Source: CAD feature listing. Evaluate the final solid. Frame: model axes, mm. A direction names the side the tool comes from. Coordinates: 2 decimals unless noted, no trailing zeros. Write each loop counter-clockwise with the first axis right and the second up, starting at its lowest first coordinate (ties: lowest second). Pieces come first, ordered by that corner, then holes. Notation, with made-up numbers: (-28, 4) - (-10, 4) arc R34 ccw to (-10, 35) - close; hole circle Ø9 at (81.5, 82.25). An arc over 180 degrees is marked (long way). One line per question, with ' | ' between items.
from build123d import *

# Parameters (mm, degrees)
F0_W     = 60
F0_H     = 20
F0_R     = 2.5
F1_DEPTH = 4
F2_W     = 20
F2_H     = 69
F2_R     = 2.5
F3_DEPTH = 4
F5_DEPTH = 60
F7_DEPTH = 65


with BuildPart() as f1:
    # F0 (on Top) → F1 (new body)
    with BuildSketch(Plane.XY):
        with Locations((30, 10)):
            Rectangle(F0_W, F0_H)
        with Locations((10, 10)):
            Circle(F0_R, mode=Mode.SUBTRACT)
        with Locations((30, 10)):
            Circle(F0_R, mode=Mode.SUBTRACT)
        with Locations((50, 10)):
            Circle(F0_R, mode=Mode.SUBTRACT)
    extrude(amount=F1_DEPTH)

    # F2 (on Right) → F3 (join)
    with BuildSketch(Plane.YZ):
        with Locations((10, 34.5)):
            Rectangle(F2_W, F2_H)
        with Locations((10, 14)):
            Circle(F2_R, mode=Mode.SUBTRACT)
        with Locations((10, 34)):
            Circle(F2_R, mode=Mode.SUBTRACT)
        with Locations((10, 54)):
            Circle(F2_R, mode=Mode.SUBTRACT)
    extrude(amount=-F3_DEPTH)

    # F4 (on face) → F5 (join, through all)
    with BuildSketch(Plane.YZ.offset(60)):
        Polygon((7, 5.5), (5.5, 4), (14.5, 4), (13, 5.5), align=None)
    extrude(amount=-F5_DEPTH)

    # F6 (on face) → F7 (join, through all)
    with BuildSketch(Plane.XY.offset(69)):
        Polygon((1.5, 13), (0, 14.5), (0, 5.5), (1.5, 7), align=None)
    extrude(amount=-F7_DEPTH)


solid = f1.part
Item 1: Cut plane A-A on x = 13.5. Return loops of the section in (y, z), and give its area (4 significant figures).
Check sheet entries:
outline: (0, 0) - (20, 0) - (20, 4) - (14.5, 4) - (13, 5.5) - (7, 5.5) - (5.5, 4) - (0, 4) - close | area: 91.25 mm²
Item 2: Pin query (flat end, axial travel): pin 1 Ø3 at (x, y) = (10, 10) entering from -Z; pin 2 Ø3 at (y, z) = (3, 27) entering from +X; pin 3 Ø8 at (x, y) = (30, 10) entering from +Z. Return the tip coordinate at first contact, or that it passes through.
Check sheet entries:
pin 1: z = 4 | pin 2: x = 0 | pin 3: z = 5.5
Item 3: Cut plane C-C on y = 15.75. Return loops of the section in (x, z), and give its area (3 significant figures).
Check sheet entries:
outline: (-4, 0) - (60, 0) - (60, 4) - (0, 4) - (0, 69) - (-4, 69) - close | area: 516 mm²
Item 4: Mould query, pull axis Z, two halves, no side actions, for faces 1 (the face through (52.31, 9.04, 1.97)), 2 (the face through (30, 3, 4)), 3 (the face through (-1.97, 9.46, 11.56)). Classes: pulls with the +Z half, pulls with the -Z half, needs draft (parallel to the pull), parting line crosses it, or undercut.
Check sheet entries:
face 1: needs draft | face 2: pulls with the +Z half | face 3: undercut
Item 5: Cut plane B-B on z = 30. Return loops of the section in (x, y).
Check sheet entries:
outline: (-4, 0) - (0, 0) - (0, 5.5) - (1.5, 7) - (1.5, 13) - (0, 14.5) - (0, 20) - (-4, 20) - close
Item 6: Access query for faces 4 (the face through (9.46, 7.56, 1.97)), 5 (the face through (31, 10, 5.5)), 6 (the face through (0.8, 13.7, 37)). Directions: +Z, -Z, +X, -X, +Y, -Y. A direction counts if a zero-diameter tool reaches every point of the face in a straight line with its end or side. Return the directions, or none.
Check sheet entries:
face 4: -Z | face 5: +Z, +X, +Y, -Y | face 6: +Z, +X, +Y
Item 7: Cut plane D-D on z = 14. Return loops of the section in (x, y), and give its area (4 significant figures).
Check sheet entries:
outline: (-4, 0) - (0, 0) - (0, 5.5) - (1.5, 7) - (1.5, 13) - (0, 14.5) - (0, 20) - (-4, 20) - (-4, 12.5) - (0, 12.5) - (0, 7.5) - (-4, 7.5) - close | area: 71.25 mm²
Item 8: Ray query, line 1 along Z through (x, y) = (-2.7, 10); line 2 along Y through (x, z) = (10, 1.35); line 3 along Z through (x, y) = (33.5, 3). Return the intervals inside material, ascending. Write a range as [from, to].
Check sheet entries:
line 1: [0, 11.5], [16.5, 31.5], [36.5, 51.5], [56.5, 69] | line 2: [0, 7.5], [12.5, 20] | line 3: [0, 4]
